Geometry: final body of the model. Coordinates: model frame, mm. Face numbers are marked on the shaded views. A direction names the side the tool comes from. Round coordinates to 2 decimals unless told otherwise and drop trailing zeros. Order: outer loops, then holes, each group sorted by start corner. A loop starts at its lowest first (then second) coordinate and runs counter-clockwise, first axis right, second up. Notation, with made-up numbers: M 8,36 L 39,36 A17 ccw 39,62 Z; hole C 18.25,65 d10. An arc over 180 degrees is marked long. Put each result on its own line as item: value. Start each with the question number.
1) Section A-A, the plane x = 0. Return loops of the section in (y, z).
2) Access query for the marked faces 4, 5 and 6. Directions: +Z, -Z, +X, -X, +Y, -Y. A direction counts if a zero-diameter tool reaches every point of the face in a straight line with its end or side. Return the directions, or none.
3) Material intervals for probe 1 along Y at (x, z) = (-67, 6); probe 2 along Z at (x, y) = (-27, -4); probe 3 along Y at (x, z) = (-59, 5), sorted ascending. Write a range as [from, to].
4) Section B-B, the plane x = -58.5. Return loops of the section in (y, z).
5) Draft query along Y for the marked faces 1, 2 and 3. Return one class per face: pulls with the +Y half, pulls with the -Y half, needs draft (parallel to the pull), parting line crosses it, or undercut.
6) First-contact query: P1, Ø17, axis at x = -2, y = 1, coming from the -Z side; P2, Ø6, axis at y = -2.5, z = -4, coming from the -X side; P3, Ø5, axis at x = -53, y = -5, coming from the -Z side; P4, Ø1, axis at x = -36.5, z = -15.5, coming from the -Y side (3 decimals). Flat tips, straight axial feed; report the tip coordinate or a pass-through.
from build123d import *

# Parameters (mm, degrees)
SZKIC1_R                         = 11
DODANIE_WYCI_GNI_CIE1_DEPTH      = 12
SZKIC4_R                         = 11.147474951019817
SZKIC4_R_2                       = 9.147474951019817
DODANIE_WYCI_GNI_CIE2_DEPTH      = 1
SZKIC13_R                        = 4.000000000000003
DODANIE_WYCI_GNI_CIE3_DEPTH      = 11.5
WYTNIJ_WYCI_GNI_CIE1_DEPTH       = 60.02626138756585
WYTNIJ_WYCI_GNI_CIE2_DEPTH       = 58.227067591020045
WYTNIJ_WYCI_GNI_CIE3_DEPTH       = 23
DODANIE_WYCI_GNI_CIE4_DEPTH      = 2.5
DODANIE_WYCI_GNI_CIE4_DEPTH_BACK = 14.5
DODANIE_WYCI_GNI_CIE5_DEPTH      = 2.5
OTWORY_USTALAJ_CE_8_0MM1_D       = 8
OTWORY_USTALAJ_CE_8_0MM1_DEPTH   = 40
OTWORY_USTALAJ_CE_8_0MM1_TIP     = 2.403442476110241
OTWORY_USTALAJ_CE_8_0MM2_D       = 8
OTWORY_USTALAJ_CE_8_0MM2_DEPTH   = 40
OTWORY_USTALAJ_CE_8_0MM2_TIP     = 2.403442476110241
SFAZOWANIE1_SIZE                 = 1
ZAOKR_GLENIE2_R                  = 2
ZAOKR_GLENIE3_R                  = 5
SFAZOWANIE2_SIZE                 = 0.5
ZAOKR_GLENIE4_R                  = 0.3
ZAOKR_GLENIE5_R                  = 5
WYTNIJ_WYCI_GNI_CIE4_START       = -3
WYTNIJ_WYCI_GNI_CIE4_DEPTH       = 3
ZAOKR_GLENIE11_R                 = 5


with BuildPart() as part:
    # Szkic1 → Dodanie-wyciągnięcie1 (new body)
    with BuildSketch(Plane.XY):
        with BuildLine():
            Line((-40, -8.000000000000005), (-2.1326786841408407, -13.836606579295779))
            ThreePointArc((-2.1326786841408407, -13.836606579295779), (12.103611293588447, -7.035807960264275), (10.968141143659846, 8.700567789101818))
            Line((10.968141143659846, 8.700567789101818), (-12.843130370941623, 38.71761875780841))
            Line((-12.843130370941623, 38.71761875780841), (-26.746589095410883, 30.799674864537906))
            Line((-26.746589095410883, 30.799674864537906), (-40, 7.999999999999995))
            Line((-40, 7.999999999999995), (-40, -8.000000000000005))
        make_face()
        Circle(SZKIC1_R, mode=Mode.SUBTRACT)
    extrude(amount=DODANIE_WYCI_GNI_CIE1_DEPTH)

    # Szkic4 → Dodanie-wyciągnięcie2 (add)
    with BuildSketch(Plane.XY.offset(12)):
        Circle(SZKIC4_R)
        Circle(SZKIC4_R_2, mode=Mode.SUBTRACT)
    extrude(amount=-DODANIE_WYCI_GNI_CIE2_DEPTH)

    # Szkic13 → Dodanie-wyciągnięcie3 (add, symmetric)
    with BuildSketch(Plane(origin=(0.996619630552348, 2.0368751739166404, 3.1e-16), x_dir=(0.8982426752029381, -0.43949982530630105, 0), z_dir=(0.4394998253063011, 0.8982426752029382, 0))):
        with BuildLine():
            Line((-36.22413445269548, 11.122577076374291), (-36.22413445269548, 8.67e-15))
            Line((-36.22413445269548, 8.67e-15), (-33.72413445269548, 7.61e-15))
            Line((-33.72413445269548, 7.61e-15), (-13.224134452695484, 6.94e-15))
            ThreePointArc((-13.224134452695484, 6.94e-15), (-17.80107386619313, 7.230855656561982), (-20.374424199879662, 15.392443491106029))
            ThreePointArc((-20.374424199879662, 15.392443491106029), (-29.935182038237862, 19.329968170654332), (-36.22413445269548, 11.122577076374291))
        make_face()
        with Locations(Location((-27.724134452695484, 11.122577076374293, 0), (0, 0, 180))):
            Circle(SZKIC13_R, mode=Mode.SUBTRACT)
    extrude(amount=DODANIE_WYCI_GNI_CIE3_DEPTH, both=True)

    # Szkic15 → Wytnij-wyciągnięcie1 (cut, through all)
    with BuildSketch(Plane(origin=(0, 0, 0), x_dir=(-1, 0, 0), z_dir=(0, 0, -1))):
        Polygon((12.843130370941623, 38.71761875780841), (26.746589095410883, 30.799674864537906), (40, 7.999999999999995), (40, -8.000000000000005), (38.494484112785884, -8.232049789295985), (38.494484112785884, 7.999999999999995), (26.00155220007409, 29.491432489730776), (12.09809347560483, 37.40937638300129), (11.896450058886177, 37.52421120875695), align=None)
    extrude(amount=-WYTNIJ_WYCI_GNI_CIE1_DEPTH, mode=Mode.SUBTRACT)

    # Szkic16 → Wytnij-wyciągnięcie2 (cut, through all)
    with BuildSketch(Plane(origin=(0, 0, 0), x_dir=(-1, 0, 0), z_dir=(0, 0, -1))):
        Polygon((26.48719581612529, 28.287166702582056), (36.59569179817021, 7.627585172914479), (36.59569179817021, -8.524716482663612), (38.494484112785884, -8.232049789295985), (38.494484112785884, 7.999999999999995), (26.00155220007409, 29.491432489730776), (11.896450058886177, 37.52421120875695), (11.389545957202317, 36.88519593201458), align=None)
    extrude(amount=-WYTNIJ_WYCI_GNI_CIE2_DEPTH, mode=Mode.SUBTRACT)

    # Szkic17 → Wytnij-wyciągnięcie3 (cut)
    with BuildSketch(Plane(origin=(-32.53806343770011, 15.920500763831628, 0), x_dir=(0, 0, 1), z_dir=(-0.898242675202938, 0.4394998253063012, 0))):
        Polygon((-27.81416800588854, 10.767622358797922), (-27.814168005888536, -7.232377641202076), (1.18e-15, -7.232377641202076), (2.5, -7.232377641202076), (2.5000000000000004, 10.767622358797922), (4.3e-16, 10.767622358797922), align=None)
    extrude(amount=-WYTNIJ_WYCI_GNI_CIE3_DEPTH, mode=Mode.SUBTRACT)

    # Szkic18 → Obrót1 (revolve)
    with BuildSketch(Plane(origin=(0, 0, 6), x_dir=(-1, 0, 0), z_dir=(0, 0, -1)), mode=Mode.PRIVATE) as obr_t1_sk:
        Polygon((76.59569179817022, 0), (76.59569179817021, -7), (74.59569179817021, -7), (74.59569179817021, -6.95), (36.59569179817021, -6.949999999999999), (36.59569179817021, 0), align=None)
    revolve(obr_t1_sk.sketch.rotate(Axis((0, 0, 6), (-1, 0, 0)), 270), axis=Axis((0, 0, 6), (-1, 0, 0)))

    # Szkic19 → Obrót2 (revolve)
    with BuildSketch(Plane(origin=(0, 0, 6), x_dir=(-1, 0, 0), z_dir=(0, 0, -1))):
        Polygon((38.44574931620652, 67.5085471625366), (32.36298612425123, 70.97264761584243), (31.373243137592404, 69.23471527528378), (31.416691446106377, 69.20997170061732), (12.611574699588953, 36.18925723000281), (18.65088517799791, 32.74989261638888), align=None)
    revolve(axis=Axis((0, 0, 6), (-0.4948714933294059, 0.868966170279329, 0)))

    # Szkic20 → Dodanie-wyciągnięcie4 (add, two sides: drawn at the far end of the back side and taken through both)
    with BuildSketch(Plane(origin=(0, 0, 0), x_dir=(-1, 0, 0), z_dir=(0, 0, -1)).offset(-DODANIE_WYCI_GNI_CIE4_DEPTH_BACK)):
        Polygon((36.59569179817021, -8.524716482663612), (34.59569179817021, -8.832982627533559), (34.59569179817021, 6.649008141474715), (36.59569179817021, 7.627585172914479), align=None)
        Polygon((26.48719581612529, 28.287166702582056), (11.389545957202317, 36.88519593201458), (10.13193011920909, 35.29981571891061), (24.31339302460761, 27.223549961252633), align=None)
    extrude(amount=DODANIE_WYCI_GNI_CIE4_DEPTH + DODANIE_WYCI_GNI_CIE4_DEPTH_BACK)

    # Szkic21 → Dodanie-wyciągnięcie5 (add)
    with BuildSketch(Plane.XY.offset(12)):
        Polygon((-24.313393024607603, 27.22354996125263), (-26.48719581612529, 28.287166702582056), (-36.59569179817021, 7.627585172914479), (-34.59569179817021, 6.649008141474715), align=None)
    extrude(amount=DODANIE_WYCI_GNI_CIE5_DEPTH)

    # Otwory ustalające Ø8.0mm1
    with Locations(Plane(origin=(-76.595691798, 0, 6), x_dir=(0, 0, -1), z_dir=(-1, 0, 0))):
        with Locations((0, 0)):
            Hole(OTWORY_USTALAJ_CE_8_0MM1_D / 2, depth=OTWORY_USTALAJ_CE_8_0MM1_DEPTH)
            with Locations((0, 0, -(OTWORY_USTALAJ_CE_8_0MM1_DEPTH + OTWORY_USTALAJ_CE_8_0MM1_TIP / 2))):  # 118° drill point
                Cone(0, OTWORY_USTALAJ_CE_8_0MM1_D / 2, OTWORY_USTALAJ_CE_8_0MM1_TIP, mode=Mode.SUBTRACT)

    # Otwory ustalające Ø8.0mm2
    with Locations(Plane(origin=(-38.445749316, 67.508547163, 6), x_dir=(0.868966170279, 0.494871493329, 0), z_dir=(-0.494871493329, 0.868966170279, 0))):
        with Locations((0, 0)):
            Hole(OTWORY_USTALAJ_CE_8_0MM2_D / 2, depth=OTWORY_USTALAJ_CE_8_0MM2_DEPTH)
            with Locations((0, 0, -(OTWORY_USTALAJ_CE_8_0MM2_DEPTH + OTWORY_USTALAJ_CE_8_0MM2_TIP / 2))):  # 118° drill point
                Cone(0, OTWORY_USTALAJ_CE_8_0MM2_D / 2, OTWORY_USTALAJ_CE_8_0MM2_TIP, mode=Mode.SUBTRACT)

    # Sfazowanie1
    sfazowanie1_edges = [part.edges().sort_by_distance(p)[0] for p in [
        (-76.59569179817021, -2.41e-15, 13),
        (-44.52851250816182, 64.04444670923077, 5.999999999999999),
    ]]
    chamfer(sfazowanie1_edges, length=SFAZOWANIE1_SIZE)

    # Zaokrąglenie2
    zaokr_glenie2_edges = [part.edges().sort_by_distance(p)[0] for p in [
        (-35.59569179817021, -8.678849555098585, 14.5),
        (-35.59569179817021, -8.678849555098585, -2.5),
        (-10.760738038205703, 36.092505825462595, 14.5),
        (-10.760738038205703, 36.092505825462595, -2.5),
    ]]
    fillet(zaokr_glenie2_edges, radius=ZAOKR_GLENIE2_R)

    # Zaokrąglenie3
    zaokr_glenie3_edges = [part.edges().sort_by_distance(p)[0] for p in [
        (-7.146113762376627, 15.483942694928315, 1.249999999999997),
        (-15.057110617890048, -0.6844254587245677, 1.2499999999999964),
        (-34.59569179817021, 6.649008141474715, -1.250000000000004),
        (-24.31339302460761, 27.223549961252633, -1.2500000000000024),
    ]]
    fillet(zaokr_glenie3_edges, radius=ZAOKR_GLENIE3_R)

    # Sfazowanie2
    sfazowanie2_edges = [part.edges().sort_by_distance(p)[0] for p in [
        (-18.364185241155525, -11.334794603414672, 12),
        (-18.364185241155525, -11.334794603414672, 0),
        (12.103611293588445, -7.0358079602642745, 12),
        (0.41810551222537384, 22.000191754006217, 0),
        (12.103611293588445, -7.0358079602642745, 0),
        (0.41810551222537384, 22.000191754006217, 12),
    ]]
    chamfer(sfazowanie2_edges, length=SFAZOWANIE2_SIZE)

    # Zaokrąglenie4
    zaokr_glenie4_edges = [part.edges().sort_by_distance(p)[0] for p in [
        (-11, -6.23e-15, 11),
    ]]
    fillet(zaokr_glenie4_edges, radius=ZAOKR_GLENIE4_R)

    # Zaokrąglenie5
    zaokr_glenie5_edges = [part.edges().sort_by_distance(p)[0] for p in [
        (-12.909559415404027, 19.973857802509606, -15.392443491106027),
        (-21.9193058341832, 1.5598829608493752, -15.39244349110603),
    ]]
    fillet(zaokr_glenie5_edges, radius=ZAOKR_GLENIE5_R)

    # Szkic29 → Wytnij-wyciągnięcie4 (cut)
    with BuildSketch(Plane.XY.offset(12).offset(WYTNIJ_WYCI_GNI_CIE4_START)):
        with BuildLine():
            Line((-29.59569179817021, -4.544604097780221), (-29.595691798170208, 5.469178555653164))
            Line((-29.595691798170208, 5.469178555653164), (-20.51960657313938, 23.630126718567237))
            Line((-20.51960657313938, 23.630126718567237), (-11.384028520269917, 28.832788580533173))
            Line((-11.384028520269917, 28.832788580533173), (0.386433954908492, 13.99466572657217))
            ThreePointArc((0.386433954908492, 13.99466572657217), (-12.103611293588447, 7.035807960264281), (-11.969655932420048, -7.261359160617354))
            Line((-11.969655932420048, -7.261359160617354), (-29.59569179817021, -4.544604097780221))
        make_face()
    extrude(amount=WYTNIJ_WYCI_GNI_CIE4_DEPTH, mode=Mode.SUBTRACT)

    # Zaokrąglenie11
    zaokr_glenie11_edges = [part.edges().sort_by_distance(p)[0] for p in [
        (0.386433954908492, 13.99466572657217, 10.5),
        (-11.96965593242005, -7.261359160617353, 10.5),
        (-29.59569179817021, -4.544604097780221, 10.5),
        (-29.595691798170208, 5.469178555653164, 10.5),
        (-20.51960657313938, 23.630126718567237, 10.5),
        (-11.384028520269917, 28.832788580533173, 10.5),
    ]]
    fillet(zaokr_glenie11_edges, radius=ZAOKR_GLENIE11_R)


solid = part.part
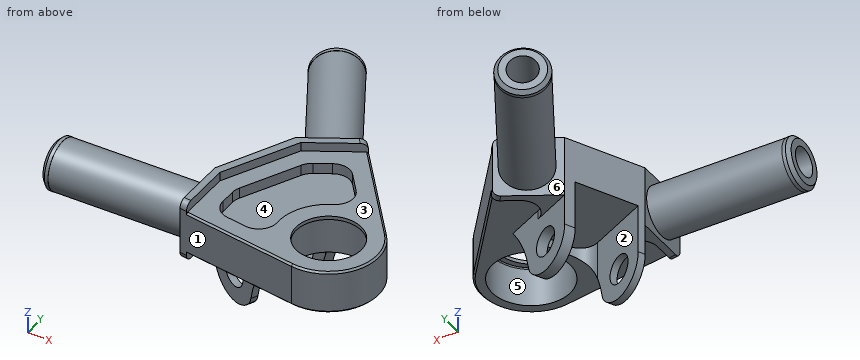
Result sheet:
1. outline: M -14,0.5 L -13.5,0 L -11,0 L -11,10.7 A0.3 cw -10.7,11 L -9.15,11 L -9.15,12 L -13.5,12 L -14,11.5 Z; M 9.15,11 L 10.7,11 A0.3 cw 11,10.7 L 11,0 L 21.72,0 L 22.53,0.5 L 22.53,11.5 L 21.72,12 L 9.15,12 Z
2. face 4: +Z
2. face 5: -Z
2. face 6: none
3. probe 1: y = [-6.95, -4], [4, 6.95]
3. probe 2: z = [0, 9]
3. probe 3: y = [-6.88, -3.87], [3.87, 6.88]
4. outline: C 0,6 d13.9; hole C 0,6 d8
5. face 1: pulls with the -Y half
5. face 2: undercut
5. face 3: needs draft
6. P1: stops at z = 11
6. P2: stops at x = -36.6
6. P3: stops at z = -0.48
6. P4: passes through
